Geometry check sheet. Reference: drawing and pictorial views, mm from the part's lowest x, y, z. Give positions to 0.01 mm unless a question says otherwise; leave off trailing zeros. Order: outer loops, then holes, each group sorted by start corner. A loop starts at its lowest first (then second) coordinate and runs counter-clockwise, first axis right, second up. Notation, with made-up numbers: M 72,-19 L 108,-19 A24 cw 108,20 Z; hole C 3.5,47.5 d4. An arc over 180 degrees is marked long. Answer as CSV lines item,"result". Start each with the question number.
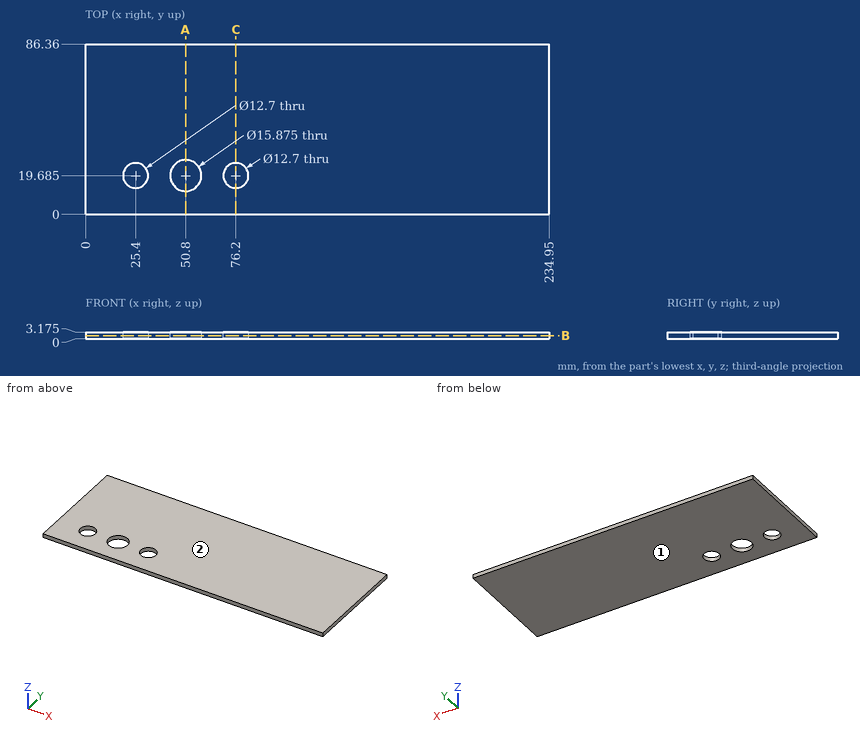
Item 1: Draft check along Z on the marked faces 1 and 2. Enter one of: pulls with the +Z half, pulls with the -Z half, needs draft (parallel to the pull), parting line crosses it, or undercut.
Item 2: Section check C-C on x = 76.2. Record the boundary of the cut face in (y, z) (3 decimals).
Item 3: Section check B-B on z = 1.6. Give the number of separate pieces and of enclosed holes in the cut face, then the cut area to 3 significant figures.
Item 4: Section check A-A on x = 50.8. Record the boundary of the cut face in (y, z) (1 decimal), then the cut area to 3 significant figures.
Item 5: Scan lines: line 1 along Y through (x, z) = (25.4, 0.6) (3 decimals); line 2 along Y through (x, z) = (50.8, 1.95); line 3 along X through (y, z) = (26.5, 0.2). Record each from-to range of solid material in increasing order.
Numbers:
1,face 1,"pulls with the -Z half"
1,face 2,"pulls with the +Z half"
2,outline,"M 0,0 L 13.335,0 L 13.335,3.175 L 0,3.175 Z; M 26.035,0 L 86.36,0 L 86.36,3.175 L 26.035,3.175 Z"
3,separate pieces,"1"
3,enclosed holes,"3"
3,area,"19,800 mm2"
4,outline,"M 0,0 L 11.7,0 L 11.7,3.2 L 0,3.2 Z; M 27.6,0 L 86.4,0 L 86.4,3.2 L 27.6,3.2 Z"
4,area,"224 mm2"
5,line 1,"0 to 13.335, 26.035 to 86.36"
5,line 2,"0 to 11.75, 27.62 to 86.36"
5,line 3,"0 to 46.73, 54.87 to 234.95"
